Work out the finished part from the listing and answer in its coordinate system (mm). Coordinates: 2 decimals unless noted, no trailing zeros. Write each loop counter-clockwise with the first axis right and the second up, starting at its lowest first coordinate (ties: lowest second). Pieces come first, ordered by that corner, then holes. Notation, with made-up numbers: (48.25, -39) - (62.25, -39) arc R25 ccw to (62.25, -9) - close; hole circle Ø2 at (-13.75, 66). An arc over 180 degrees is marked (long way). Use a Markdown table: item, result. Add a question column.
(1) Given pin 1 Ø1.5 at (y, z) = (2, -3) entering from +X; pin 2 Ø1 at (x, y) = (1, 1) entering from -Z, each flat-ended and moving along its own axis, determine where each tip first touches the part or whether it passes through.
(2) Find the intervals of material crossed by line 1 (X direction, y = 2.25, z = 0); line 2 (Z direction, x = -1, y = 2.3); line 3 (Z direction, x = 1.5, y = 1.85), in increasing order. Write a range as from..to.
(3) The part is cut by section A-A, the plane y = 2.25. Give the vertices of the cut face in (x, z).
(4) The part is cut by section B-B, the plane z = 0. Give the vertices of the cut face in (x, y), then the cut area to 3 significant figures.
(5) For a pull along Z with two mould halves and no side action, classify faces 1 (the face through (-3, 1.2, 1.8)), 2 (the face through (-2, 1, 0)), 3 (the face through (3, 1.2, -1.8)), 4 (the face through (-2, 0, -1)) as released by +Z, released by -Z, zero draft, split by the parting line, or undercut.
(6) The part is cut by section D-D, the plane x = -3. Give the vertices of the cut face in (y, z), then the cut area to 3 significant figures.
(7) The part is cut by section C-C, the plane x = 1.75. Give the vertices of the cut face in (y, z).
from build123d import *

# Parameters (mm, degrees)
BOSS_EXTRUDE1_DEPTH = 2.5
SKETCH2_R           = 2
CUT_EXTRUDE1_DEPTH  = 6.912925747
FILLET1_R           = 0.25


with BuildPart() as part:
    # Sketch1 → Boss-Extrude1 (new body)
    with BuildSketch(Plane(origin=(0, 0, 0), x_dir=(1, 0, 0), z_dir=(0, 1, 0))):
        Polygon((1.98810578, 3.518631658), (-2.053171512, 3.481065939), (-4.041277292, -0.037565718), (-1.98810578, -3.518631658), (2.053171512, -3.481065939), (4.041277292, 0.037565718), align=None)
    extrude(amount=BOSS_EXTRUDE1_DEPTH)

    # Sketch2 → Cut-Extrude1 (cut, through all)
    with BuildSketch(Plane(origin=(0, 2.5, 0), x_dir=(1, 0, 0), z_dir=(0, 1, 0))):
        with Locations(Location((0, 0, 0), (0, 0, 270))):
            Circle(SKETCH2_R)
    extrude(amount=-CUT_EXTRUDE1_DEPTH, mode=Mode.SUBTRACT)

    # Fillet1
    fillet1_edges = [part.edges().sort_by_distance(p)[0] for p in [
        (4.041277292, 1.25, -0.037565718),
        (2.053171512, 1.25, 3.481065939),
        (-1.98810578, 1.25, 3.518631658),
        (-4.041277292, 1.25, 0.037565718),
        (-2.053171512, 1.25, -3.481065939),
        (1.98810578, 1.25, -3.518631658),
    ]]
    fillet(fillet1_edges, radius=FILLET1_R)


solid = part.part
Model answer:
| question | item | result |
|---|---|---|
| 1 | pin 1 | x = 2.74 |
| 1 | pin 2 | z = -3.51 |
| 2 | line 1 | -4..-2, 2..4 |
| 2 | line 2 | -3.49..-1.73, 1.73..3.51 |
| 2 | line 3 | -3.51..-1.32, 1.32..3.49 |
| 3 | outline | (-3.97, -0.09) - (-2.12, -3.36) arc R0.25 ccw to (-1.91, -3.48) - (1.84, -3.52) arc R0.25 ccw to (2.06, -3.39) - (3.97, -0.16) arc R0.25 ccw to (3.97, 0.09) - (2.12, 3.36) arc R0.25 ccw to (1.91, 3.48) - (-1.84, 3.52) arc R0.25 ccw to (-2.06, 3.39) - (-3.97, 0.16) arc R0.25 ccw to start; hole circle Ø4 at (0, 0) |
| 4 | outline | (-4, 0) - (-2, 0) - (-2, 2.5) - (-4, 2.5) - close; (2, 0) - (4, 0) - (4, 2.5) - (2, 2.5) - close |
| 4 | area | 10.0 mm^2 |
| 5 | face 1 | released by +Z |
| 5 | face 2 | undercut |
| 5 | face 3 | released by -Z |
| 5 | face 4 | zero draft |
| 6 | outline | (0, -1.81) - (2.5, -1.81) - (2.5, 1.8) - (0, 1.8) - close |
| 6 | area | 9.02 mm^2 |
| 7 | outline | (0, -3.52) - (2.5, -3.52) - (2.5, -0.97) - (0, -0.97) - close; (0, 0.97) - (2.5, 0.97) - (2.5, 3.48) - (0, 3.48) - close |
